from build123d import *

# Parameters (mm, degrees)
ESQUISSE2_R      = 2
EXTRUSION1_DEPTH = 45


with BuildPart() as part:
    # Esquisse1 → Révolution1 (revolve)
    with BuildSketch(Plane.XY):
        Polygon((0, 10), (0, 17.5), (5, 17.5), (5, 11), (44, 11), (44, 6.5), (20, 6.5), (20, 10), align=None)
    revolve(axis=Axis((0, 0, 0), (1, 0, 0)))

    # Esquisse2 → Extrusion1 (cut, through all)
    with BuildSketch(Plane.ZY):
        with Locations((0, 15)):
            Circle(ESQUISSE2_R)
        with Locations((15, 0)):
            Circle(ESQUISSE2_R)
        with Locations((0, -15)):
            Circle(ESQUISSE2_R)
        with Locations((-15, 0)):
            Circle(ESQUISSE2_R)
    extrude(amount=-EXTRUSION1_DEPTH, mode=Mode.SUBTRACT)


solid = part.part
Verification items for the finished model (mm, model axes). A direction names the side the tool comes from. Give positions to 0.01 mm unless a question says otherwise; leave off trailing zeros. Write each loop counter-clockwise with the first axis right and the second up, starting at its lowest first coordinate (ties: lowest second). Pieces come first, ordered by that corner, then holes. Notation, with made-up numbers: (56, -14.75) - (115, -14.75) arc R19 cw to (115, -4.75) - close; hole circle Ø7 at (76.25, 29.5). An arc over 180 degrees is marked (long way). Answer as CSV lines item,"result". Start each with the question number.
1. Set-up check for faces 5 (the face through (5, -8, -8)), 6 (the face through (31.832, -5.158, -3.955)), 7 (the face through (20, -7, 0)): record each of +Z, -Z, +X, -X, +Y, -Y from which the full face is reachable in a straight line by a thin tool's end or side.
2. Sectioned sample at C-C (z = 14.5). Record the boundary of the cut face in (x, y), then the cut area to 3 significant figures.
3. Draft check along Y on faces 1 (the face through (0, -8, -8)), 2 (the face through (2.535, -13.887, -10.648)), 3 (the face through (2.5, -1.2, 13.4)), 4 (the face through (2.5, -1.2, -16.6)). Enter one of: pulls with the +Y half, pulls with the -Y half, needs draft (parallel to the pull), parting line crosses it, or undercut.
4. Depth check by flat-ended pin: pin 1 (6.5 mm diameter, centred on y = 15, z = 0, fed in from +X); pin 2 (3 mm diameter, centred on x = 21, z = -0.5, fed in from -Y); pin 3 (6 mm diameter, centred on y = 3, z = 4, fed in from -X). Enter the tip coordinate at first touch or a pass-through.
5. Thickness scan on line 1 (X direction, y = -11.5, z = -5.5); line 2 (Z direction, x = 25.75, y = 0); line 3 (X direction, y = -2.5, z = 8.5). Record the ranges inside material, lowest first.
6. Sectioned sample at A-A (y = 0). Record the boundary of the cut face in (x, z), then the cut area to 3 significant figures.
7. Sectioned sample at D-D (y = -15). Record the boundary of the cut face in (x, z), then the cut area to 3 significant figures.
Derived:
1,face 5,"+X"
1,face 6,"+X, -X"
1,face 7,"-X"
2,outline,"(0, -9.8) - (5, -9.8) - (5, -1.94) - (0, -1.94) - close; (0, 1.94) - (5, 1.94) - (5, 9.8) - (0, 9.8) - close"
2,area,"78.6 mm²"
3,face 1,"needs draft"
3,face 2,"parting line crosses it"
3,face 3,"undercut"
3,face 4,"undercut"
4,pin 1,"x = 5"
4,pin 2,"y = -11"
4,pin 3,"x = 20"
5,line 1,"0 to 5"
5,line 2,"-11 to -6.5, 6.5 to 11"
5,line 3,"20 to 44"
6,outline,"(0, -17.5) - (5, -17.5) - (5, -17) - (0, -17) - close; (0, -13) - (5, -13) - (5, -11) - (44, -11) - (44, -6.5) - (20, -6.5) - (20, -10) - (0, -10) - close; (0, 10) - (20, 10) - (20, 6.5) - (44, 6.5) - (44, 11) - (5, 11) - (5, 13) - (0, 13) - close; (0, 17) - (5, 17) - (5, 17.5) - (0, 17.5) - close"
6,area,"281 mm²"
7,outline,"(0, -9.01) - (5, -9.01) - (5, -2) - (0, -2) - close; (0, 2) - (5, 2) - (5, 9.01) - (0, 9.01) - close"
7,area,"70.1 mm²"
